Geometry: final body of the model. Coordinates: model frame, mm. Round coordinates to 2 decimals unless told otherwise and drop trailing zeros. Write each loop counter-clockwise with the first axis right and the second up, starting at its lowest first coordinate (ties: lowest second). Pieces come first, ordered by that corner, then holes. Notation, with made-up numbers: M 17,-12 L 66,-12 A12 ccw 66,6 Z; hole C 79.25,44 d10. An arc over 180 degrees is marked long. Answer as CSV lines item,"result". Start each with the question number.
Q1. Section query A-A on y = -16. Output: boundary loops of the cut face in (x, z).
Q2. Section query B-B on x = 12. Output: boundary loops of the cut face in (y, z).
Q3. First-contact query: pin 1 (5 mm diameter, centred on x = 0, z = 5, fed in from -Y); pin 2 (4 mm diameter, centred on x = -40, z = 7, fed in from -Y); pin 3 (10 mm diameter, centred on y = -10.5, z = 1.5, fed in from +X). Flat tips, straight axial feed; report the tip coordinate or a pass-through.
Q4. Ray query, probe 1 along Z at (x, y) = (-90, -2.25); probe 2 along Y at (x, z) = (-62, -1); probe 3 along X at (y, z) = (8, -0.5). Return the intervals inside material, ascending.
Q5. Section query C-C on y = 19.5. Output: boundary loops of the cut face in (x, z), and give its area (3 significant figures).
```python
from build123d import *

# Parameters (mm, degrees)
F0_W     = 240
F0_H     = 20
F1_DEPTH = 4
F3_DEPTH = 20
F4_R     = 5
F5_R     = 3.25
F6_DEPTH = 25
F7_SIZE  = 3
F8_R     = 1.55
F9_DEPTH = 25


with BuildPart() as f1:
    # F0 (on Front) → F1 (new body)
    with BuildSketch(Plane.XZ):
        Rectangle(F0_W, F0_H)
    extrude(amount=F1_DEPTH)

    # F2 (on face) → F3 (join)
    with BuildSketch(Plane.XZ.offset(4)):
        Polygon((5.370641, 3.310112), (2.399305, 5.83472), (-1.488484, 6.130664), (-4.807723, 4.084902), (-6.290574, 0.478847), (-5.370641, -3.310112), (-2.399305, -5.83472), (1.488484, -6.130664), (4.807723, -4.084902), (6.290574, -0.478847), align=None)
    extrude(amount=F3_DEPTH)

    # F4
    f4_edges = [f1.edges().sort_by_distance(p)[0] for p in [
        (5.549149, -24, -2.281874),
        (5.830608, -24, 1.415633),
        (3.884973, -24, 4.572416),
        (0.45541, -24, 5.982692),
        (-3.148103, -24, 5.107783),
        (-5.549149, -24, 2.281874),
        (-5.830608, -24, -1.415633),
        (-3.884973, -24, -4.572416),
        (-0.45541, -24, -5.982692),
        (3.148103, -24, -5.107783),
    ]]
    fillet(f4_edges, radius=F4_R)

    # F5 (on face) → F6 (join)
    with BuildSketch(Plane(origin=(0, 0, 0), x_dir=(-1, 0, 0), z_dir=(0, 1, 0))):
        Circle(F5_R)
    extrude(amount=F6_DEPTH)

    # F7
    f7_edges = [f1.edges().sort_by_distance(p)[0] for p in [
        (3.25, 25, 0),
    ]]
    chamfer(f7_edges, length=F7_SIZE)

    # F8 (on face) → F9 (cut)
    with BuildSketch(Plane(origin=(0, 0, 0), x_dir=(-1, 0, 0), z_dir=(0, 1, 0))):
        with Locations((-90, 0)):
            Circle(F8_R)
        with Locations((90, 0)):
            Circle(F8_R)
    extrude(amount=-F9_DEPTH, mode=Mode.SUBTRACT)


solid = f1.part
```
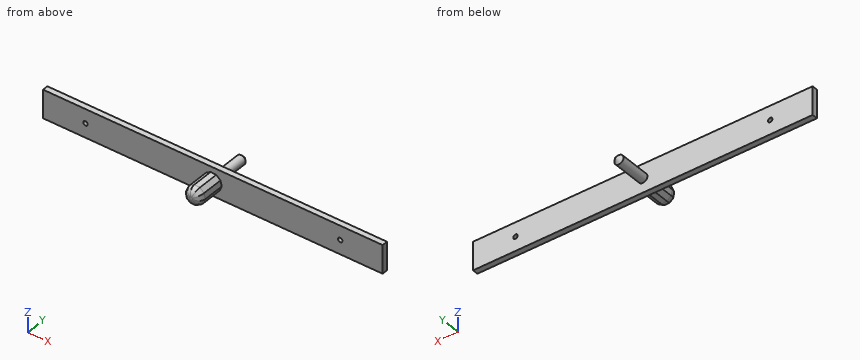
Entries:
1,outline,"M -6.29,0.48 L -5.37,-3.31 L -2.4,-5.83 L 1.49,-6.13 L 4.81,-4.08 L 6.29,-0.48 L 5.37,3.31 L 2.4,5.83 L -1.49,6.13 L -4.81,4.08 Z"
2,outline,"M -4,-10 L 0,-10 L 0,10 L -4,10 Z"
3,pin 1,"stops at y = -23.77"
3,pin 2,"stops at y = -4"
3,pin 3,"stops at x = 6.29"
4,probe 1,"z = -10 to -1.55, 1.55 to 10"
4,probe 2,"y = -4 to 0"
4,probe 3,"x = -3.21 to 3.21"
5,outline,"C 0,0 d6.5"
5,area,"33.2 mm^2"
